Autodesk Inventor part; units mm, degrees
ref_plane "YZ Plane" through (0, 0, 0) normal (1, 0, 0) x (0, 1, 0)
ref_plane "XZ Plane" through (0, 0, 0) normal (0, 1, 0) x (-1, 0, 0)
ref_plane "XY Plane" through (0, 0, 0) normal (0, 0, 1) x (1, 0, 0)
sketch "Sketch1" plane through (0, 0, 0) normal (0, 0, 1) x (1, 0, 0)
  arc A0 (-50.8, 107.95) -> (-53.975, 104.775) centre (-50.8, 104.775) ccw
  line L0 (-53.975, 104.775) -> (-53.975, 39.4462)
  arc A1 (-53.975, 39.4462) -> (-50.8, 36.2712) centre (-50.8, 39.4462) ccw
  line L1 (-50.8, 36.2712) -> (-42.4561, 36.2712)
  arc A2 (-39.2811, 33.0962) -> (-42.4561, 36.2712) centre (-42.4561, 33.0962) ccw
  line L2 (-39.2811, 33.0962) -> (-39.2811, 3.175)
  arc A3 (-39.2811, 3.175) -> (-36.1061, 0) centre (-36.1061, 3.175) ccw
  line L3 (-36.1061, 0) -> (36.1061, 0)
  arc A4 (36.1061, 0) -> (39.2811, 3.175) centre (36.1061, 3.175) ccw
  line L4 (39.2811, 3.175) -> (39.2811, 33.0962)
  arc A5 (42.4561, 36.2712) -> (39.2811, 33.0962) centre (42.4561, 33.0962) ccw
  line L5 (42.4561, 36.2712) -> (50.8, 36.2712)
  arc A6 (50.8, 36.2712) -> (53.975, 39.4462) centre (50.8, 39.4462) ccw
  line L6 (53.975, 39.4462) -> (53.975, 104.775)
  arc A7 (53.975, 104.775) -> (50.8, 107.95) centre (50.8, 104.775) ccw
  line L7 (50.8, 107.95) -> (-50.8, 107.95)
  arc A8 (39.4081, 39.3192) -> (36.2331, 36.1442) centre (39.4081, 36.1442) ccw
  line L8 (36.2331, 36.1442) -> (36.2331, 9.271)
  arc A9 (33.0581, 6.096) -> (36.2331, 9.271) centre (33.0581, 9.271) ccw
  line L9 (33.0581, 6.096) -> (-33.0581, 6.096)
  arc A10 (-36.2331, 9.271) -> (-33.0581, 6.096) centre (-33.0581, 9.271) ccw
  line L10 (-36.2331, 9.271) -> (-36.2331, 36.1442)
  arc A11 (-36.2331, 36.1442) -> (-39.4081, 39.3192) centre (-39.4081, 36.1442) ccw
  line L11 (-39.4081, 39.3192) -> (-47.752, 39.3192)
  arc A12 (-50.927, 42.4942) -> (-47.752, 39.3192) centre (-47.752, 42.4942) ccw
  line L12 (-50.927, 42.4942) -> (-50.927, 98.679)
  arc A13 (-47.752, 101.854) -> (-50.927, 98.679) centre (-47.752, 98.679) ccw
  line L13 (-47.752, 101.854) -> (47.752, 101.854)
  arc A14 (50.927, 98.679) -> (47.752, 101.854) centre (47.752, 98.679) ccw
  line L14 (50.927, 98.679) -> (50.927, 42.4942)
  arc A15 (47.752, 39.3192) -> (50.927, 42.4942) centre (47.752, 42.4942) ccw
  line L15 (47.752, 39.3192) -> (39.4081, 39.3192)
  circle A16 centre (-50.927, 104.902) radius 1.5
  circle A17 centre (36.2331, 3.048) radius 1.5
  circle A18 centre (-36.2331, 3.048) radius 1.5
  circle A19 centre (50.927, 104.902) radius 1.5
  line L16 (0, 0) -> (0, -19.0308)
extrude "Extrusion1" add sketch "Sketch1" along normal blind 3 contours L7 A7 L6 A6 L5 A5 L4 A4 L3 A3 L2 A2 L1 A1 L0 A0 | A8 L8 A9 L9 A10 L10 A11 L11 A12 L12 A13 L13 A14 L14 A15 L15
fillet "Fillet1" radius 1.25 16 edges at (53.0451, 107.0201, 3) (0, 107.95, 3) (-53.0451, 107.0201, 3) (-53.975, 72.1106, 3) (-53.0451, 37.2011, 3) (-46.6281, 36.2712, 3) (-40.211, 35.3413, 3) (-39.2811, 18.1356, 3) (-38.3512, 0.9299, 3) (0, 0, 3) (38.3512, 0.9299, 3) (39.2811, 18.1356, 3) (40.211, 35.3413, 3) (46.6281, 36.2712, 3) (53.0451, 37.2011, 3) (53.975, 72.1106, 3)
sketch "Sketch2" plane through (0, 0, 3) normal (0, 0, 1) x (1, 0, 0)
  arc A0 (-30.9142, 9.83) -> (-32.3284, 10.83) centre (-32.3284, 9.33) ccw
  line L0 (-32.5, 10.83) -> (-32.3284, 10.83)
  line L1 (-32.5, 80.83) -> (-32.5, 10.83)
  line L2 (32.5, 80.83) -> (-32.5, 80.83)
  line L3 (32.5, 10.83) -> (32.5, 80.83)
  line L4 (32.3284, 10.83) -> (32.5, 10.83)
  arc A1 (32.3284, 10.83) -> (30.9142, 9.83) centre (32.3284, 9.33) ccw
  arc A2 (29.5, 8.83) -> (30.9142, 9.83) centre (29.5, 10.33) ccw
  line L5 (29.5, 8.83) -> (-29.5, 8.83)
  arc A3 (-30.9142, 9.83) -> (-29.5, 8.83) centre (-29.5, 10.33) ccw
  arc A4 (-35, 85.33) -> (-37, 83.33) centre (-35, 83.33) ccw
  line L6 (-37, 8.33) -> (-37, 83.33)
  arc A5 (-37, 8.33) -> (-35, 6.33) centre (-35, 8.33) ccw
  line L7 (35, 6.33) -> (-35, 6.33)
  arc A6 (35, 6.33) -> (37, 8.33) centre (35, 8.33) ccw
  line L8 (37, 83.33) -> (37, 8.33)
  arc A7 (37, 83.33) -> (35, 85.33) centre (35, 83.33) ccw
  line L9 (-35, 85.33) -> (35, 85.33)
  circle A8 centre (34, 82.33) radius 1.5
  circle A9 centre (-34, 82.33) radius 1.5
  circle A10 centre (-34, 9.33) radius 1.5
  circle A11 centre (34, 9.33) radius 1.5
  line L10 (36.1061, 1.25) -> (-36.1061, 1.25)
  line L11 (0, 6.33) -> (0, -2.8147)
  line L12 (0, 1.25) -> (0, 6.33)
  line L13 (0, 8.83) -> (0, 34.23)
  line L14 (0, 34.23) -> (-19.05, 34.23)
  line L15 (-19.05, 34.23) -> (-19.05, 53.28)
  line L16 (-19.05, 53.28) -> (19.05, 53.28)
  line L17 (19.05, 53.28) -> (19.05, 34.23)
  line L18 (19.05, 34.23) -> (0, 34.23)
  point P0 (0, 0)
  point P1 (0, 67.33)
  dimension "d4" = 5.08
  dimension "d5" = 25.4
  dimension "d6" = 19.05
  dimension "d7" = 19.05
  dimension "d8" = 38.1
  dimension "d9" = 19.05
extrude "Extrusion2" cut sketch "Sketch2" against normal through all contours L14 L15 L16 L17 L18 | A8 | A9 | A10 | A11
fillet "Fillet2" radius 3.175 4 edges at (-19.05, 53.28, 1.5) (-19.05, 34.23, 1.5) (19.05, 34.23, 1.5) (19.05, 53.28, 1.5)
properties part number "bit bot lid 1"
The listing builds one solid part. Answer for the finished solid, in the listing's coordinates (mm). A direction names the side the tool comes from. Round coordinates to 2 decimals unless told otherwise and drop trailing zeros. Write each loop counter-clockwise with the first axis right and the second up, starting at its lowest first coordinate (ties: lowest second). Pieces come first, ordered by that corner, then holes. Notation, with made-up numbers: M 69.5,20.25 L 112.5,20.25 A29 cw 112.5,42.25 Z; hole C -30.5,-24.75 d6. An arc over 180 degrees is marked long. Write each question's results on one line, items separated by ' | '. Start each with the question number.
Item 1: For a pull along X with two mould halves and no side action, classify faces 1 (the face through (-18.14, 52.33, 1.48)), 2 (the face through (-1, 55, 0)), 3 (the face through (40.19, 35.32, 0.86)) as pulls with the +X half, pulls with the -X half, needs draft (parallel to the pull), parting line crosses it, or undercut.
Item 2: Straight lines are drawn through the part: L1, parallel to X at y = 82.33, z = 1.2 (3 decimals); L2, parallel to Y at x = 34, z = 0.7; L3, parallel to X at y = 82.33, z = 2.2. For each, find the intervals that lie inside material, in ascending order. Write a range as [from, to].
Item 3: For faces 4 (the face through (-53.07, 106.995, 0.863)), 5 (the face through (18.1, 52.37, 1.48)), determine the directions among +Z, -Z, +X, -X, +Y, -Y from which every point of the face is accessible in a straight line to the end or side of a thin tool.
Item 4: A cutting plane is placed at B-B on y = 82.33. Write down the section's boundary in (x, z) (3 decimals).
Item 5: Flat-ended cylindrical pins translate along their axes: pin 1 Ø1.8 at (x, y) = (34, 9.33) entering from -Z; pin 2 Ø1.4 at (x, z) = (48.5, 1) entering from -Y. Find the tip coordinate at first contact, or state that the pin passes through.
Item 6: A cutting plane is placed at C-C on y = 16.5. Write down the section's boundary in (x, z), and give its area (3 significant figures).
Item 7: A cutting plane is placed at A-A on y = 42.5. Write down the section's boundary in (x, z) (3 decimals), and give its area (3 significant figures).
Check sheet entries:
1) face 1: undercut | face 2: needs draft | face 3: pulls with the +X half
2) L1: [-53.975, -35.5], [-32.5, 32.5], [35.5, 53.975] | L2: [0, 7.83], [10.83, 80.83], [83.83, 107.95] | L3: [-53.89, -35.5], [-32.5, 32.5], [35.5, 53.89]
3) face 4: +Z, -Z, -X, +Y | face 5: +Z, -Z
4) outline: M -53.975,0 L -35.5,0 L -35.5,3 L -52.725,3 A1.25 ccw -53.975,1.75 Z; M -32.5,0 L 32.5,0 L 32.5,3 L -32.5,3 Z; M 35.5,0 L 53.975,0 L 53.975,1.75 A1.25 ccw 52.725,3 L 35.5,3 Z
5) pin 1: through | pin 2: y = 36.27
6) outline: M -39.28,0 L 39.28,0 L 39.28,1.75 A1.25 ccw 38.03,3 L -38.03,3 A1.25 ccw -39.28,1.75 Z | area: 235 mm²
7) outline: M -53.975,0 L -19.05,0 L -19.05,3 L -52.725,3 A1.25 ccw -53.975,1.75 Z; M 19.05,0 L 53.975,0 L 53.975,1.75 A1.25 ccw 52.725,3 L 19.05,3 Z | area: 209 mm²
